Can you work these out from the model? Positions are in its coordinate system, mm. Face numbers are marked on the shaded views. A direction names the side the tool comes from. Round coordinates to 2 decimals unless told otherwise and drop trailing zeros. Order: outer loops, then holes, each group sorted by start corner. A loop starts at its lowest first (then second) coordinate and runs counter-clockwise, first axis right, second up.
Q1. Will these pins go through, and if not, where does the flat tip stop? P1, Ø5, axis at y = -1.5, z = 2, coming from the -X side; P2, Ø1, axis at x = 35.5, z = 4, coming from the +Y side (3 decimals).
Q2. If we section it at A-A (y = 0): Please give me the cut outline in (x, z).
Q3. If we section it at C-C (z = -10.5): Please give me the cut outline in (x, y), plus the area to 3 significant figures.
Q4. If we section it at D-D (y = 5): Please give me the cut outline in (x, z), plus the area to 3 significant figures.
Q5. For the marked faces 1 and 2, which set-ups out of +Z, -Z, +X, -X, +Y, -Y let a thin tool reach every point of the face, with its end or its side?
Q6. If we section it at B-B (x = 21): Please give me the cut outline in (y, z).
Q7. We'd pull the mould along Y, two halves only. Please class the marked faces 3, 4 and 5: pulls with the +Y half, pulls with the -Y half, needs draft (parallel to the pull), parting line crosses it, or undercut.
Q8. If I drill on line 1 (Z direction, x = -15, y = 2.25); line 2 (Y direction, x = -27, z = -7.75); line 3 (X direction, y = 0, z = -9.25), over which ranges is the centre line in solid material (lowest first)?
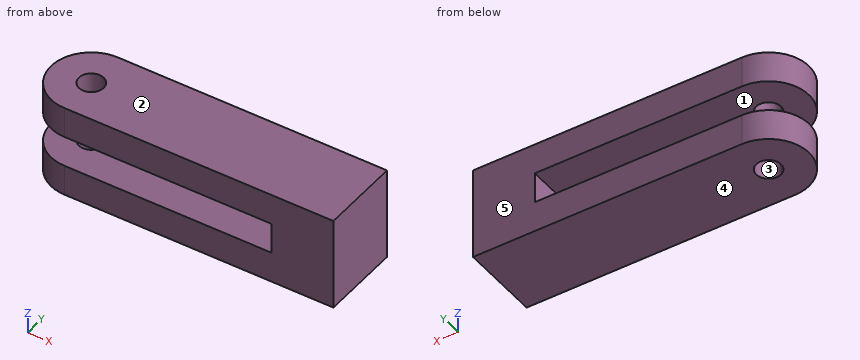
from build123d import *

# Parameters (mm, degrees)
SKETCH_1_W                = 120
SKETCH_1_H                = 26
EXTRUDE_1_DEPTH           = 15
CUT_EXTRUDE_START         = -15
CUT_EXTRUDE_8_DEPTH       = 15
CUT_EXTRUDE_9_DEPTH       = 64.198101237
CUT_EXTRUDE_9_DEPTH_BACK  = 5
CUT_EXTRUDE_10_DEPTH      = 63.20128616
CUT_EXTRUDE_10_DEPTH_BACK = 63.20128616
SKETCH_7_R                = 4


# Read off the part's stored shape, not the designer's step: 切除-拉伸8
with BuildPart() as part:
    # 草图1 → 凸台-拉伸1 (new body)
    with BuildSketch(Plane.XY):
        Rectangle(SKETCH_1_W, SKETCH_1_H)
    extrude(amount=EXTRUDE_1_DEPTH)

    # 切除-拉伸8 outline → 切除-拉伸8 (cut)
    with BuildSketch(Plane(origin=(0, 0, 0), x_dir=(-1, 0, 0), z_dir=(0, 0, -1)).offset(CUT_EXTRUDE_START)):
        with BuildLine():
            Line((60, 13), (27, 13))
            ThreePointArc((27, 13), (40, 0), (27, -13))
            Line((27, -13), (60, -13))
            Line((60, -13), (60, 13))
        make_face()
    extrude(amount=CUT_EXTRUDE_8_DEPTH, mode=Mode.SUBTRACT)

    # 草图6 → 切除-拉伸9 (cut, two sides: drawn at the far end of the back side and taken through both)
    with BuildSketch(Plane(origin=(0, 0, 0), x_dir=(-1, 0, 0), z_dir=(0, 0, -1)).offset(-CUT_EXTRUDE_9_DEPTH_BACK)):
        Polygon((-40, 191.237926759), (-40, 13), (-40, -13), (-40, -191.237926759), (316.475853517, -191.237926759), (316.475853517, 191.237926759), align=None)
    extrude(amount=CUT_EXTRUDE_9_DEPTH + CUT_EXTRUDE_9_DEPTH_BACK, mode=Mode.SUBTRACT)

    # 草图7 → 切除-拉伸10 (cut, two sides: drawn at the far end of the back side and taken through both)
    with BuildSketch(Plane(origin=(0, 0, 5), x_dir=(-1, 0, 0), z_dir=(0, 0, -1)).offset(-CUT_EXTRUDE_10_DEPTH_BACK)):
        with Locations((27, 0)):
            Circle(SKETCH_7_R)
    extrude(amount=CUT_EXTRUDE_10_DEPTH + CUT_EXTRUDE_10_DEPTH_BACK, mode=Mode.SUBTRACT)

    # 镜向2: part across plane


with BuildPart() as part_1:
    add(part.part)
    add(part.part.mirror(Plane(origin=(0, 0, 0), x_dir=(1, 0, 0), z_dir=(0, 0, -1))))


solid = part_1.part
Solution:
1. P1: stops at x = 40
1. P2: passes through
2. outline: (-40, -15) - (-31, -15) - (-31, -5) - (-40, -5) - close; (-40, 5) - (-31, 5) - (-31, 15) - (-40, 15) - close; (-23, -15) - (60, -15) - (60, 15) - (-23, 15) - (-23, 5) - (40, 5) - (40, -5) - (-23, -5) - close
3. outline: (-27, -13) - (60, -13) - (60, 13) - (-27, 13) arc R13 ccw to start; hole circle Ø8 at (-27, 0)
3. area: 2,480 mm2
4. outline: (-39, -15) - (60, -15) - (60, 15) - (-39, 15) - (-39, 5) - (40, 5) - (40, -5) - (-39, -5) - close
4. area: 2,180 mm2
5. face 1: -X, +Y, -Y
5. face 2: +Z, +X, -X, +Y, -Y
6. outline: (-13, -15) - (13, -15) - (13, -5) - (-13, -5) - close; (-13, 5) - (13, 5) - (13, 15) - (-13, 15) - close
7. face 3: undercut
7. face 4: needs draft
7. face 5: pulls with the +Y half
8. line 1: z = -15 to -5, 5 to 15
8. line 2: y = -13 to -4, 4 to 13
8. line 3: x = -40 to -31, -23 to 60
